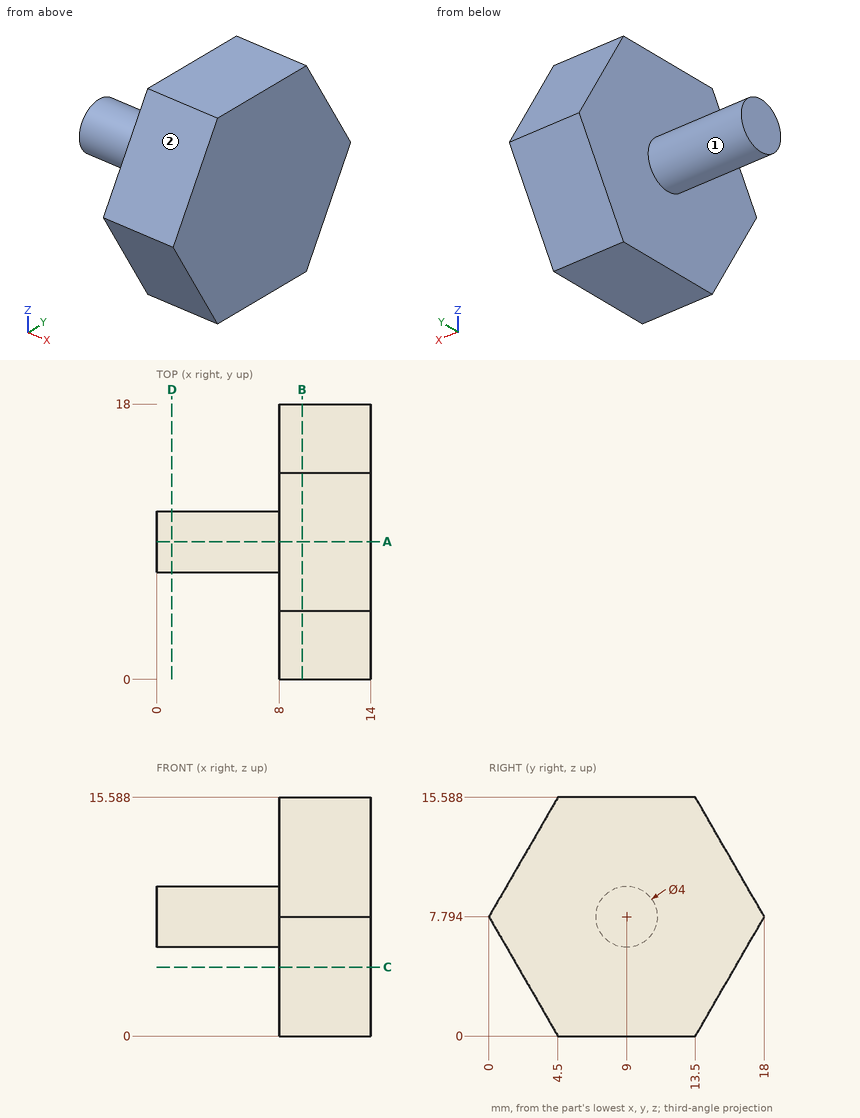
The drawing under review shows one solid part. Ordinate dimensions are in mm from its lowest x, y, z. A direction names the side the tool comes from. Round coordinates to 2 decimals unless told otherwise and drop trailing zeros. Write each loop counter-clockwise with the first axis right and the second up, starting at its lowest first coordinate (ties: lowest second). Pieces come first, ordered by that corner, then holes. Notation, with made-up numbers: (-38.75, 27.25) - (18.25, 27.25) arc R24 ccw to (18.25, 46.25) - close; hole circle Ø6 at (-36.75, 52). An arc over 180 degrees is marked (long way). Use one line per item in the form item = value.
Q1. Consider section C-C (z = 4.5). State the section outline as (x, y) points.
Answer key:
outline = (8, 1.9) - (14, 1.9) - (14, 16.1) - (8, 16.1) - close
Q2. For line 1 (X direction, y = 2.5, z = 7.25); line 2 (Y direction, x = 12, z = 12.5) (1 decimal); line 3 (Z direction, x = 6.75, y = 8.25), list the stretches that pass through material, from the lowest coordinate up. Write a range as [from, to].
Answer key:
line_1 = [8, 14]
line_2 = [2.7, 15.3]
line_3 = [5.94, 9.65]
Q3. Consider section A-A (y = 9). State the section outline as (x, z) points (1 decimal).
Answer key:
outline = (0, 5.8) - (8, 5.8) - (8, 0) - (14, 0) - (14, 15.6) - (8, 15.6) - (8, 9.8) - (0, 9.8) - close
Q4. Consider section B-B (x = 9.5). State the section outline as (y, z) points (1 decimal).
Answer key:
outline = (0, 7.8) - (4.5, 0) - (13.5, 0) - (18, 7.8) - (13.5, 15.6) - (4.5, 15.6) - close
Q5. Tool access review of the marked faces 1 and 2: name each direction out of +Z, -Z, +X, -X, +Y, -Y from which nothing blocks a thin tool from reaching the whole face with its end or side.
Answer key:
face_1 = -X
face_2 = +Z, +X, -X, -Y
Q6. Insertion check: pin 1 Ø1.5 at (x, z) = (3.5, 8) entering from +Y; pin 2 Ø1 at (y, z) = (8, 12) entering from -X; pin 3 Ø8 at (x, z) = (3.5, 9.5) entering from -Y. Each pin has a flat end and moves straight along its axis. Give the tip position at first contact, or say it passes through.
Answer key:
pin_1 = 11
pin_2 = 8
pin_3 = 7
Q7. Consider section D-D (x = 1). State the section outline as (y, z) points (1 decimal).
Answer key:
outline = circle Ø4 at (9, 7.8)
